For this review, take the finished solid that the model builds, in its own axes (mm). Face numbers are marked on the shaded views. Round coordinates to 2 decimals unless told otherwise and drop trailing zeros. Write each loop counter-clockwise with the first axis right and the second up, starting at its lowest first coordinate (ties: lowest second). Pieces come first, ordered by that corner, then holes. Notation, with made-up numbers: M 18,-18 L 62,-18 A25 cw 62,1 Z; hole C -26.75,-2 d6. An arc over 180 degrees is marked long. Use one line per item in the form item = value. Start each with the question number.
Item 1: For line 1 (Z direction, x = -5, y = 1.15); line 2 (X direction, y = 1.65, z = 1.75); line 3 (X direction, y = 1.1, z = -0.5), list the stretches that pass through material, from the lowest coordinate up. Write a range as [from, to].
Item 2: Add section A-A (z = 0). State the section outline as (x, y) points.
Item 3: For P1, Ø3.5, axis at x = -5, z = 0, coming from the -Y side, flat-tipped, find the tip position at first contact; note if it passes through.
Item 4: Add section D-D (z = 2.75). State the section outline as (x, y) points, and give its area (3 significant figures).
Item 5: Draft analysis for pull direction X (two halves, no side actions). For the marked faces 1, 2 and 3, state which applies: released by +X, released by -X, zero draft, split by the parting line, or undercut.
Item 6: Add section B-B (y = 1.65). State the section outline as (x, z) points, and give its area (3 significant figures).
Item 7: Add section C-C (x = 4.25). State the section outline as (y, z) points.
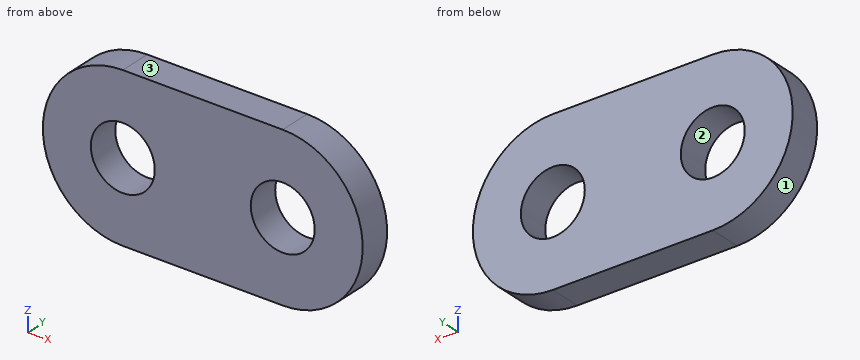
Autodesk Inventor part; units mm, degrees
ref_plane "YZ Plane" through (0, 0, 0) normal (1, 0, 0) x (0, 1, 0)
ref_plane "XZ Plane" through (0, 0, 0) normal (0, 1, 0) x (-1, 0, 0)
ref_plane "XY Plane" through (0, 0, 0) normal (0, 0, 1) x (1, 0, 0)
sketch "Sketch1" plane through (0, 0, 0) normal (0, 1, 0) x (-1, 0, 0)
  arc A0 (5, -5) -> (5, 5) centre (5, 0) ccw
  arc A1 (-5, 5) -> (-5, -5) centre (-5, 0) ccw
  line L0 (0, -7) -> (0, 7)
  line L1 (5, -5) -> (-5, -5)
  line L2 (5, 5) -> (-5, 5)
  circle A2 centre (5, 0) radius 2
  circle A3 centre (-5, 0) radius 2
  point P0 (0, 0)
  point P1 (-10, 0)
  point P2 (10, 0)
  dimension "d0" = 10
  dimension "d1" = 4
  dimension "d3" = 20
extrude "Extrusion1" add sketch "Sketch1" along normal blind 2
properties part number "T Slot Nut"
Calculated:
q1.line_1 = [-5, -2], [2, 5]
q1.line_2 = [-9.68, -5.97], [-4.03, 4.03], [5.97, 9.68]
q1.line_3 = [-9.97, -6.94], [-3.06, 3.06], [6.94, 9.97]
q2.outline = M -10,0 L -7,0 L -7,2 L -10,2 Z; M -3,0 L 3,0 L 3,2 L -3,2 Z; M 7,0 L 10,0 L 10,2 L 7,2 Z
q3.P1 = through
q4.outline = M -9.18,0 L 9.18,0 L 9.18,2 L -9.18,2 Z
q4.area = 36.7 mm^2
q5.face_1 = released by -X
q5.face_2 = undercut
q5.face_3 = zero draft
q6.outline = M -5,-5 L 5,-5 A5 ccw 5,5 L -5,5 A5 ccw Z; hole C -5,0 d4; hole C 5,0 d4
q6.area = 153 mm^2
q7.outline = M 0,-5 L 2,-5 L 2,-1.85 L 0,-1.85 Z; M 0,1.85 L 2,1.85 L 2,5 L 0,5 Z
